The figure shows three views and two pictorial views of one solid part (mm, origin at its lowest corner). Answer the questions. A direction names the side the tool comes from. Coordinates: 2 decimals unless noted, no trailing zeros. Order: outer loops, then holes, each group sorted by start corner. A loop starts at its lowest first (then second) coordinate and runs counter-clockwise, first axis right, second up. Notation, with made-up numbers: (18, 31.5) -> (41, 31.5) arc R15 ccw to (41, 54.5) -> close; hole circle Ø2 at (26, -4). An arc over 180 degrees is marked (long way). Use one line per item in the form item = value.
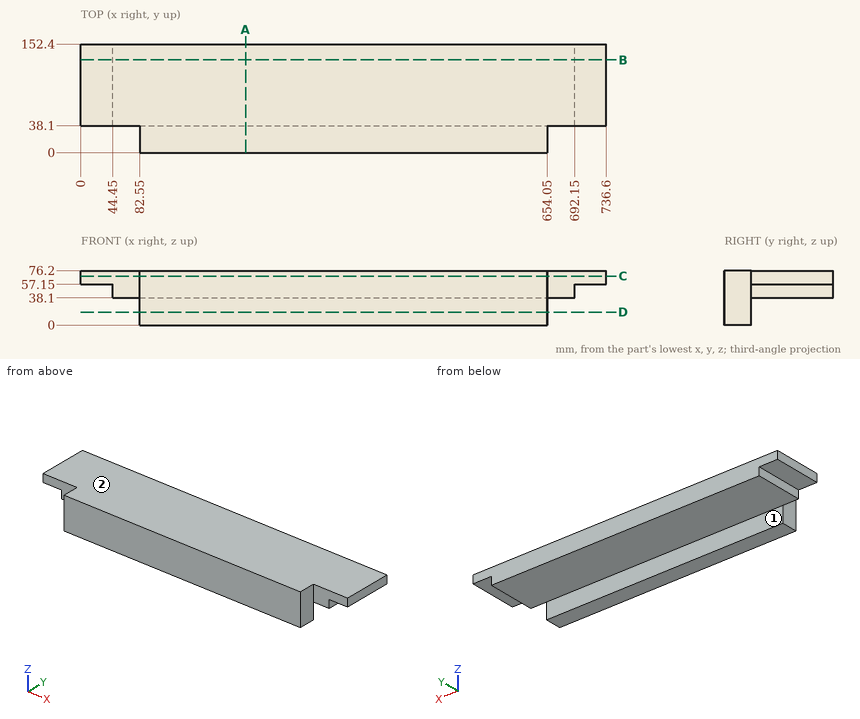
(1) Section A-A on x = 231 is taken. Write down the section's boundary in (y, z).
Data:
outline = (0, 0) -> (38.1, 0) -> (38.1, 38.1) -> (152.4, 38.1) -> (152.4, 76.2) -> (0, 76.2) -> close
(2) Section B-B on y = 130 is taken. Write down the section's boundary in (x, z), plus the area to 3 significant figures.
Data:
outline = (0, 57.15) -> (44.45, 57.15) -> (44.45, 38.1) -> (692.15, 38.1) -> (692.15, 57.15) -> (736.6, 57.15) -> (736.6, 76.2) -> (0, 76.2) -> close
area = 26,400 mm²
(3) Each of these flat-tipped pins is pushed along its axis until it touches: P1, Ø22, axis at x = 708, y = 82, coming from the -Z side; P2, Ø5, axis at x = 657, z = 45, coming from the -Y side; P3, Ø6, axis at x = 196, y = 122, coming from the -Z side. Where does it stop, or does it pass through?
Data:
P1 = 57.15
P2 = 38.1
P3 = 38.1
(4) Section D-D on z = 18 is taken. Write down the section's boundary in (x, y).
Data:
outline = (82.55, 0) -> (654.05, 0) -> (654.05, 38.1) -> (82.55, 38.1) -> close
(5) Straight lines are drawn through the part: line 1 along Y through (x, z) = (527.5, 19.5); line 2 along X through (y, z) = (29, 56); line 3 along Z through (x, y) = (655.5, 56). For each, find the intervals that lie inside material, in ascending order.
Data:
line_1 = 0 to 38.1
line_2 = 82.55 to 654.05
line_3 = 38.1 to 76.2
(6) Section C-C on z = 68.5 is taken. Write down the section's boundary in (x, y), plus the area to 3 significant figures.
Data:
outline = (0, 38.1) -> (82.55, 38.1) -> (82.55, 0) -> (654.05, 0) -> (654.05, 38.1) -> (736.6, 38.1) -> (736.6, 152.4) -> (0, 152.4) -> close
area = 106,000 mm²
(7) Which of the six approach directions +Z, -Z, +X, -X, +Y, -Y give full straight-line access (tool end or side, diameter ignored) to the marked faces 1 and 2?
Data:
face_1 = -Z, +X, -X, +Y
face_2 = +Z, +X, -X, +Y, -Y
